Work out the finished part from the listing and answer in its coordinate system (mm). A direction names the side the tool comes from. Round coordinates to 2 decimals unless told otherwise and drop trailing zeros. Loops run counter-clockwise (first coordinate to the right, second up) from the corner with the lowest first, then second, coordinate; pieces in that order, holes last. Notation, with made-up numbers: (86.25, 7.5) - (125.25, 7.5) arc R17 cw to (125.25, 18.5) - close; hole circle Ø11 at (41.5, 3). An arc over 180 degrees is marked (long way). Return JSON: item names as keys, results as strings.
from build123d import *

# Parameters (mm, degrees)
SKETCH1_R           = 1.27
SKETCH1_R_2         = 0.55
BOSS_EXTRUDE1_DEPTH = 1.57
FILLET1_R           = 0.8
SKETCH2_W           = 2.5
SKETCH2_H           = 2.5
BOSS_EXTRUDE2_DEPTH = 0.93
FILLET2_R           = 0.2


with BuildPart() as part:
    # Sketch1 → Boss-Extrude1 (new body)
    with BuildSketch(Plane.XY):
        Polygon((-9.5, 19), (-9.5, 6), (-7.6, 6), (-7.6, 0), (7.6, 0), (7.6, 6), (9.5, 6), (9.5, 19), align=None)
        with Locations((-6.75, 16.3)):
            Circle(SKETCH1_R, mode=Mode.SUBTRACT)
        with Locations((6.75, 16.3)):
            Circle(SKETCH1_R, mode=Mode.SUBTRACT)
        with Locations((0, 1.27)):
            Circle(SKETCH1_R_2, mode=Mode.SUBTRACT)
        with Locations((-5.08, 1.27)):
            Circle(SKETCH1_R_2, mode=Mode.SUBTRACT)
        with Locations((5.08, 1.27)):
            Circle(SKETCH1_R_2, mode=Mode.SUBTRACT)
        with Locations((-2.54, 1.57)):
            Circle(SKETCH1_R_2, mode=Mode.SUBTRACT)
        with Locations((2.54, 1.57)):
            Circle(SKETCH1_R_2, mode=Mode.SUBTRACT)
    extrude(amount=BOSS_EXTRUDE1_DEPTH)

    # Fillet1
    fillet1_edges = [part.edges().sort_by_distance(p)[0] for p in [
        (9.5, 6, 0.785),
        (7.6, 6, 0.785),
        (7.6, 0, 0.785),
        (-7.6, 0, 0.785),
        (-7.6, 6, 0.785),
        (-9.5, 6, 0.785),
        (-9.5, 19, 0.785),
        (9.5, 19, 0.785),
    ]]
    fillet(fillet1_edges, radius=FILLET1_R)

    # Sketch2 → Boss-Extrude2 (add)
    with BuildSketch(Plane.XY.offset(1.57)):
        with Locations((0, 16)):
            Rectangle(SKETCH2_W, SKETCH2_H)
    extrude(amount=BOSS_EXTRUDE2_DEPTH)

    # Fillet2
    fillet2_edges = [part.edges().sort_by_distance(p)[0] for p in [
        (1.25, 16, 2.5),
        (0, 17.25, 2.5),
        (-1.25, 16, 2.5),
        (0, 14.75, 2.5),
    ]]
    fillet(fillet2_edges, radius=FILLET2_R)


solid = part.part
1) A tool of negligible diameter and unlimited length cuts with its end or side. For faces 4 (the flat face through (0, 19, 1)), 5 (the flat face through (-7.6, 3, 1)), 6 (the flat face through (7.6, 3, 1)), from which of +Z, -Z, +X, -X, +Y, -Y can it reach the whole face along a straight path? Write none if from no direction.
Verdict:
{"face 4": "+Z, -Z, +X, -X, +Y", "face 5": "+Z, -Z, -X, -Y", "face 6": "+Z, -Z, +X, -Y"}
2) Find the intervals of material crossed by L1, parallel to Y at x = -6.75, z = 1.1; L2, parallel to Y at x = -2.54, z = 1.2; L3, parallel to Z at x = -3.5, y = 9.75, in increasing order.
Verdict:
{"L1": "y = 0 to 15.03, 17.57 to 19", "L2": "y = 0 to 1.02, 2.12 to 19", "L3": "z = 0 to 1.57"}
3) Flat-ended cylindrical pins translate along their axes: pin 1 (3.5 mm diameter, centred on x = 6.75, y = 16.3, fed in from +Z); pin 2 (1.5 mm diameter, centred on x = 3, y = 4.5, fed in from -Z); pin 3 (0.8 mm diameter, centred on y = 3.5, z = 1, fed in from -X); pin 4 (0.7 mm diameter, centred on x = 5.08, y = 1.27, fed in from -Z). Find the tip coordinate at first contact, or state that the pin passes through.
Verdict:
{"pin 1": "stops at z = 1.57", "pin 2": "stops at z = 0", "pin 3": "stops at x = -7.6", "pin 4": "passes through"}
4) Section A-A (x = -5.08) is taken. Give the vertices of the cut face in (y, z), and give its area (3 significant figures).
Verdict:
{"outline": "(0, 0) - (0.72, 0) - (0.72, 1.57) - (0, 1.57) - close; (1.82, 0) - (19, 0) - (19, 1.57) - (1.82, 1.57) - close", "area": "28.1 mm2"}
5) Section B-B (z = 1.05) is taken. Give the vertices of the cut face in (x, y).
Verdict:
{"outline": "(-9.5, 6.8) arc R0.8 ccw to (-8.7, 6) - (-8.4, 6) arc R0.8 cw to (-7.6, 5.2) - (-7.6, 0.8) arc R0.8 ccw to (-6.8, 0) - (6.8, 0) arc R0.8 ccw to (7.6, 0.8) - (7.6, 5.2) arc R0.8 cw to (8.4, 6) - (8.7, 6) arc R0.8 ccw to (9.5, 6.8) - (9.5, 18.2) arc R0.8 ccw to (8.7, 19) - (-8.7, 19) arc R0.8 ccw to (-9.5, 18.2) - close; hole circle Ø2.54 at (-6.75, 16.3); hole circle Ø1.1 at (-5.08, 1.27); hole circle Ø1.1 at (-2.54, 1.57); hole circle Ø1.1 at (0, 1.27); hole circle Ø1.1 at (2.54, 1.57); hole circle Ø1.1 at (5.08, 1.27); hole circle Ø2.54 at (6.75, 16.3)"}
6) Section C-C (y = 16.3) is taken. Give the vertices of the cut face in (x, z), and give its area (3 significant figures).
Verdict:
{"outline": "(-9.5, 0) - (-8.02, 0) - (-8.02, 1.57) - (-9.5, 1.57) - close; (-5.48, 0) - (5.48, 0) - (5.48, 1.57) - (1.25, 1.57) - (1.25, 2.3) arc R0.2 ccw to (1.05, 2.5) - (-1.05, 2.5) arc R0.2 ccw to (-1.25, 2.3) - (-1.25, 1.57) - (-5.48, 1.57) - close; (8.02, 0) - (9.5, 0) - (9.5, 1.57) - (8.02, 1.57) - close", "area": "24.2 mm2"}
7) Section D-D (x = 0) is taken. Give the vertices of the cut face in (y, z).
Verdict:
{"outline": "(0, 0) - (0.72, 0) - (0.72, 1.57) - (0, 1.57) - close; (1.82, 0) - (19, 0) - (19, 1.57) - (17.25, 1.57) - (17.25, 2.3) arc R0.2 ccw to (17.05, 2.5) - (14.95, 2.5) arc R0.2 ccw to (14.75, 2.3) - (14.75, 1.57) - (1.82, 1.57) - close"}
8) Determine the mould class of faces 1 (the cylindrical face through (-5.63, 1.29, 0.77)), 2 (the flat face through (0, 0, 1)), 3 (the flat face through (-9.5, 13, 1)) for opening direction X: pulls with the +X half, pulls with the -X half, needs draft (parallel to the pull), parting line crosses it, or undercut.
Verdict:
{"face 1": "undercut", "face 2": "needs draft", "face 3": "pulls with the -X half"}
